from build123d import *

# Parameters (mm, degrees)
BOSS_EXTRU_1_DEPTH      = 10
BOSS_EXTRU_1_DEPTH_BACK = 10
ESQUISSE3_R             = 1.5
BOSS_EXTRU_2_DEPTH      = 10


with BuildPart() as part:
    # Esquisse1 → Boss.-Extru.1 (new, two sides: drawn at the far end of the back side and taken through both)
    with BuildSketch(Plane.XY.offset(-BOSS_EXTRU_1_DEPTH_BACK)):
        Polygon((0, 0), (33.75, 0), (33.75, 20.85), (40.125, 20.85), (40.125, 22.65), (33.75, 22.65), (33.75, 30), (14.925, 30), (14.925, 35.25), (0, 35.25), (0, 22.65), (-6.375, 22.65), (-6.375, 20.85), (0, 20.85), align=None)
    extrude(amount=BOSS_EXTRU_1_DEPTH + BOSS_EXTRU_1_DEPTH_BACK)

    # Esquisse3 → Boss.-Extru.2 (add)
    with BuildSketch(Plane(origin=(0, 30, 0), x_dir=(1, 0, 0), z_dir=(0, 1, 0))):
        with Locations(Location((24.3375, 0, 0), (0, 0, 270))):
            Circle(ESQUISSE3_R)
    extrude(amount=BOSS_EXTRU_2_DEPTH)


solid = part.part
Work out the finished part from the listing and answer in its coordinate system (mm). A direction names the side the tool comes from. Round coordinates to 2 decimals unless told otherwise and drop trailing zeros. Write each loop counter-clockwise with the first axis right and the second up, starting at its lowest first coordinate (ties: lowest second). Pieces come first, ordered by that corner, then holes. Notation, with made-up numbers: (-34, 55) - (-24, 55) arc R34 cw to (-24, 88) - close; hole circle Ø5 at (-40, 24.25). An arc over 180 degrees is marked (long way). Answer in a Markdown table with one row per item. Add a question column.
1. Find the intervals of material crossed by line 1 along Y through (x, z) = (28, -1.5); line 2 along X through (y, z) = (33.5, 2.75) (3 decimals); line 3 along X through (y, z) = (18.5, -1.25), in increasing order. Write a range as from..to.
2. A cutting plane is placed at C-C, the plane y = 7. Determine the outline of the cut face in (x, z), and give its area (3 significant figures).
3. A cutting plane is placed at B-B, the plane x = 33. Determine the outline of the cut face in (y, z), and give its area (3 significant figures).
4. A cutting plane is placed at A-A, the plane z = 8.75. Determine the outline of the cut face in (x, y) (3 decimals).
5. Given pin 1 (12 mm diameter, centred on x = 7, z = -4, fed in from +Y); pin 2 (6 mm diameter, centred on y = 32.5, z = -1.5, fed in from -X); pin 3 (4 mm diameter, centred on y = 32.5, z = 2.5, fed in from +X), each flat-ended and moving along its own axis, determine where each tip first touches the part or whether it passes through.
6. For faces 1 (the flat face through (0, 11, 0)), 2 (the flat face through (37, 20.85, 0)), 3 (the flat face through (-3, 22.65, 0)), determine the directions among +Z, -Z, +X, -X, +Y, -Y from which every point of the face is accessible in a straight line to the end or side of a thin tool.
7. The mould has two halves that part along X. Classify faces 4 (the cylindrical face through (22.873, 34.93, -0.325)), 5 (the flat face through (33.75, 10, 0)), 6 (the flat face through (0, 29, 0)), 7 (the flat face through (17, 18, 10)): +X half, -X half, draft (parallel to the pull), parting line (faces both ways), or undercut.
Worked out:
| question | item | result |
|---|---|---|
| 1 | line 1 | 0..30 |
| 1 | line 2 | 0..14.925 |
| 1 | line 3 | 0..33.75 |
| 2 | outline | (0, -10) - (33.75, -10) - (33.75, 10) - (0, 10) - close |
| 2 | area | 675 mm^2 |
| 3 | outline | (0, -10) - (30, -10) - (30, 10) - (0, 10) - close |
| 3 | area | 600 mm^2 |
| 4 | outline | (-6.375, 20.85) - (0, 20.85) - (0, 0) - (33.75, 0) - (33.75, 20.85) - (40.125, 20.85) - (40.125, 22.65) - (33.75, 22.65) - (33.75, 30) - (14.925, 30) - (14.925, 35.25) - (0, 35.25) - (0, 22.65) - (-6.375, 22.65) - close |
| 5 | pin 1 | y = 35.25 |
| 5 | pin 2 | x = 0 |
| 5 | pin 3 | x = 25.75 |
| 6 | face 1 | +Z, -Z, -X, -Y |
| 6 | face 2 | +Z, -Z, +X, -Y |
| 6 | face 3 | +Z, -Z, -X, +Y |
| 7 | face 4 | undercut |
| 7 | face 5 | +X half |
| 7 | face 6 | -X half |
| 7 | face 7 | draft |
